Source: CAD feature listing. Evaluate the final solid. Frame: model axes, mm. Face numbers are marked on the shaded views. A direction names the side the tool comes from. Round coordinates to 2 decimals unless told otherwise and drop trailing zeros. Loops run counter-clockwise (first coordinate to the right, second up) from the corner with the lowest first, then second, coordinate; pieces in that order, holes last. Notation, with made-up numbers: M 54.5,20.5 L 84.5,20.5 A27 ccw 84.5,50.5 Z; hole C 71.25,58.25 d5. An arc over 180 degrees is marked long. One line per item, written item: value.
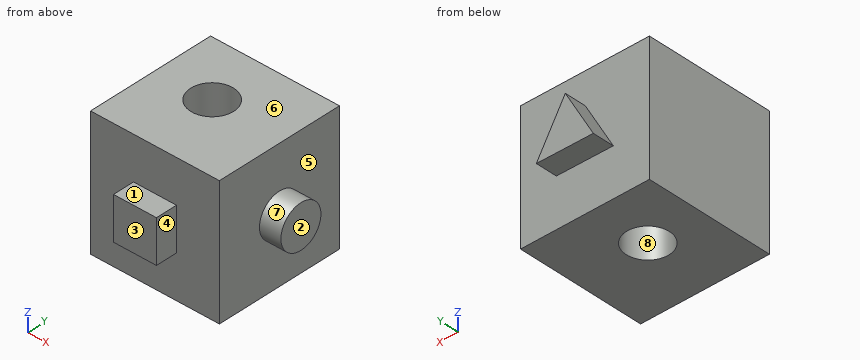
from build123d import *

# Parameters (mm, degrees)
F0_W     = 76.2
F0_H     = 76.2
F1_DEPTH = 76.2
F2_R     = 12.7
F3_DEPTH = 12.7
F4_W     = 25.4
F4_H     = 25.4
F5_DEPTH = 12.7
F7_D     = 25.4
F9_DEPTH = 12.7


with BuildPart() as f1:
    # F0 (on Front) → F1 (new body)
    with BuildSketch(Plane.XZ):
        with Locations((-49.343084, 67.806647)):
            Rectangle(F0_W, F0_H)
    extrude(amount=F1_DEPTH)

    # F2 (on face) → F3 (join)
    with BuildSketch(Plane.YZ.offset(-11.243084)):
        with Locations((-38.1, 67.806647)):
            Circle(F2_R)
    extrude(amount=F3_DEPTH)

    # F4 (on face) → F5 (join)
    with BuildSketch(Plane.XZ.offset(76.2)):
        with Locations((-49.343084, 67.806647)):
            Rectangle(F4_W, F4_H)
    extrude(amount=F5_DEPTH)

    # F7 (through all)
    with Locations(Plane.XY.offset(105.906647)):
        with Locations((-54.589249, -34.257531)):
            Hole(F7_D / 2)

    # F8 (on face) → F9 (join)
    with BuildSketch(Plane(origin=(0, 0, 0), x_dir=(-1, 0, 0), z_dir=(0, 1, 0))):
        Polygon((66.085933, 57.915788), (49.537393, 87.251809), (32.405924, 58.252343), align=None)
    extrude(amount=F9_DEPTH)


solid = f1.part
1. Reachability of the marked faces 1, 2, 3, 4 and 5 from +Z, -Z, +X, -X, +Y, -Y: full face, straight path, thin tool, end or side. Return the list, or none.
Report:
face 1: +Z, +X, -X, -Y
face 2: +Z, -Z, +X, +Y, -Y
face 3: +Z, -Z, +X, -X, -Y
face 4: +Z, -Z, +X, -Y
face 5: +X
2. Section query D-D (y = -52.5). Return the cut outline in (x, z), and give its area (3 significant figures).
Report:
outline: M -87.44,29.71 L -11.24,29.71 L -11.24,105.91 L -87.44,105.91 Z
area: 5,810 mm2
3. Section query B-B (y = -38.1). Return the cut outline in (x, z).
Report:
outline: M -87.44,29.71 L -66.69,29.71 L -66.69,105.91 L -87.44,105.91 Z; M -42.48,29.71 L -11.24,29.71 L -11.24,55.11 L 1.46,55.11 L 1.46,80.51 L -11.24,80.51 L -11.24,105.91 L -42.48,105.91 Z
4. Pull-direction query (Y, two-part tool) for the marked faces 6, 7 and 8; classes: released by +Y, released by -Y, zero draft, split by the parting line, or undercut.
Report:
face 6: zero draft
face 7: split by the parting line
face 8: undercut
5. Section query C-C (x = -75). Return the cut outline in (y, z), and give its area (3 significant figures).
Report:
outline: M -76.2,29.71 L 0,29.71 L 0,105.91 L -76.2,105.91 Z
area: 5,810 mm2
6. Ray query, line 1 (X direction, y = -35, z = 46); line 2 (Y direction, x = -27, z = 38); line 3 (X direction, y = -2, z = 85.5). Return the intervals inside material, ascending. Write a range as [from, to].
Report:
line 1: x = [-87.44, -67.27], [-41.91, -11.24]
line 2: y = [-76.2, 0]
line 3: x = [-87.44, -11.24]
7. Section query A-A (z = 71). Return the cut outline in (x, y).
Report:
outline: M -87.44,-76.2 L -62.04,-76.2 L -62.04,-88.9 L -36.64,-88.9 L -36.64,-76.2 L -11.24,-76.2 L -11.24,-50.39 L 1.46,-50.39 L 1.46,-25.81 L -11.24,-25.81 L -11.24,0 L -39.94,0 L -39.94,12.7 L -58.71,12.7 L -58.71,0 L -87.44,0 Z; hole C -54.59,-34.26 d25.4
8. Pin query (flat end, axial travel): pin 1 (23 mm diameter, centred on x = -32.5, z = 50.5, fed in from +Y); pin 2 (14 mm diameter, centred on y = -82, z = 64.5, fed in from +X); pin 3 (2 mm diameter, centred on x = -20.5, z = 59.5, fed in from +Y); pin 4 (4 mm diameter, centred on y = -81, z = 63, fed in from -X). Return the tip coordinate at first contact, or that it passes through.
Report:
pin 1: stops at y = 12.7
pin 2: stops at x = -11.24
pin 3: stops at y = 0
pin 4: stops at x = -62.04
